Could you check a few things on this drawing? It's one solid part, dimensions in mm from its lowest x, y, z. Give positions to 0.01 mm unless a question says otherwise; leave off trailing zeros. Loops run counter-clockwise (first coordinate to the right, second up) from the corner with the lowest first, then second, coordinate; pieces in that order, holes last.
1. Imagine slicing it at D-D (x = 41.5). List the corners of the cut face in (y, z) for me.
2. Imagine slicing it at C-C (x = 33). List the corners of the cut face in (y, z) for me, plus the area to 3 significant figures.
3. Imagine slicing it at A-A (y = 10). List the corners of the cut face in (x, z) for me, plus the area to 3 significant figures.
4. Thinking about a two-plate mould opening in Z: for the marked faces 1, 2 and 3, which applies, +Z half, -Z half, draft (parallel to the pull), parting line (faces both ways), or undercut?
5. I need wall thicknesses on line 1 along Z through (x, y) = (13, 1.1); line 2 along Z through (x, y) = (10, 17). Which ranges of each line are inside material? Lowest first, please.
6. For P1, Ø3, axis at x = 6.5, z = 16, coming from the +Y side; P2, Ø4.5, axis at x = 33, y = 10, coming from the -Z side; P3, Ø3, axis at x = 37, y = 6, coming from the +Z side, each with a flat end and sliding along its axis, tell me the tip position at first contact or that it passes through.
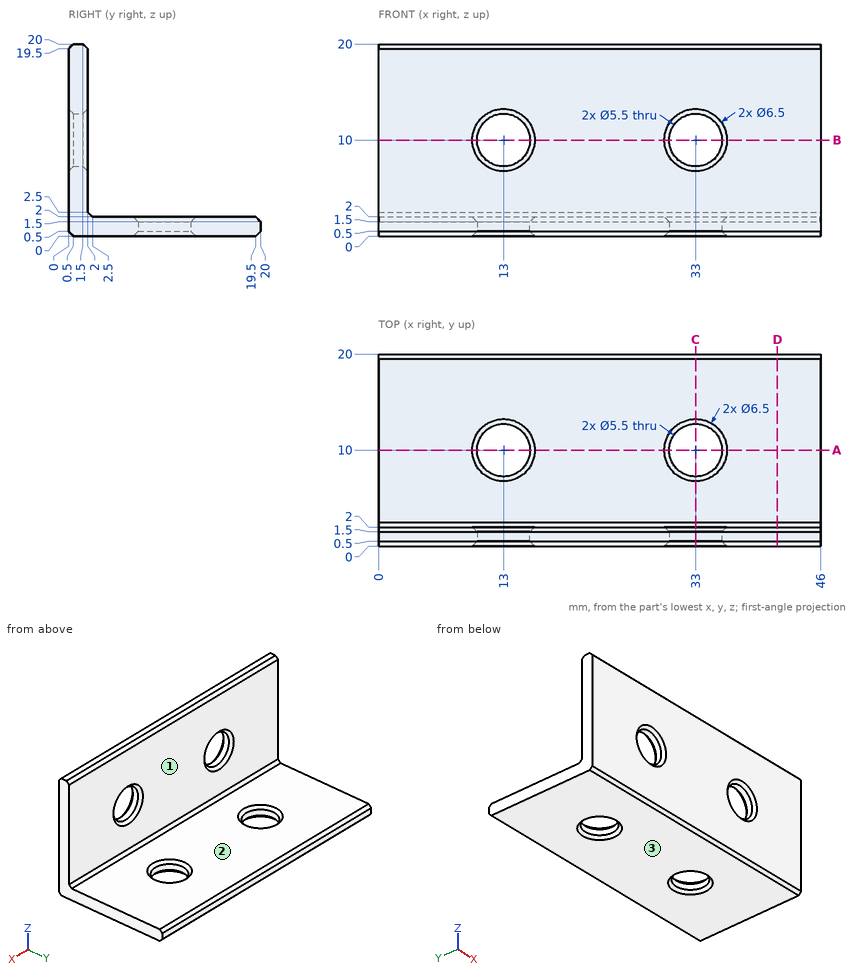
Derived:
1. outline: (0, 0.5) - (0.5, 0) - (19.5, 0) - (20, 0.5) - (20, 1.5) - (19.5, 2) - (2.5, 2) - (2, 2.5) - (2, 19.5) - (1.5, 20) - (0.5, 20) - (0, 19.5) - close
2. outline: (0, 0.5) - (0.5, 0) - (6.75, 0) - (7.25, 0.5) - (7.25, 1.5) - (6.75, 2) - (2.5, 2) - (2, 2.5) - (2, 6.75) - (1.5, 7.25) - (0.5, 7.25) - (0, 6.75) - close; (0, 13.25) - (0.5, 12.75) - (1.5, 12.75) - (2, 13.25) - (2, 19.5) - (1.5, 20) - (0.5, 20) - (0, 19.5) - close; (12.75, 0.5) - (13.25, 0) - (19.5, 0) - (20, 0.5) - (20, 1.5) - (19.5, 2) - (13.25, 2) - (12.75, 1.5) - close
2. area: 52.5 mm2
3. outline: (0, 0) - (9.75, 0) - (10.25, 0.5) - (10.25, 1.5) - (9.75, 2) - (0, 2) - close; (15.75, 0.5) - (16.25, 0) - (29.75, 0) - (30.25, 0.5) - (30.25, 1.5) - (29.75, 2) - (16.25, 2) - (15.75, 1.5) - close; (35.75, 0.5) - (36.25, 0) - (46, 0) - (46, 2) - (36.25, 2) - (35.75, 1.5) - close
3. area: 69.0 mm2
4. face 1: draft
4. face 2: +Z half
4. face 3: -Z half
5. line 1: z = 0 to 7.25, 12.75 to 20
5. line 2: z = 0 to 2
6. P1: stops at y = 2
6. P2: passes through
6. P3: stops at z = 2
